```python
from build123d import *

# Parameters (mm, degrees)
SZKIC1_W                     = 53
SZKIC1_H                     = 374
SZKIC1_W_2                   = 24
SZKIC1_H_2                   = 365
DODANIE_WYCI_GNI_CIE2_DEPTH  = 12
SZKIC2_W                     = 12
SZKIC2_H                     = 3.5
WYTNIJ_WYCI_GNI_CIE1_DEPTH   = 2
SZKIC3_W                     = 53
SZKIC3_H                     = 374
DODANIE_WYCI_GNI_CIE3_DEPTH  = 2
SZKIC4_W                     = 13.3
SZKIC4_H                     = 30.500081729
SZKIC4_W_2                   = 9.4
SZKIC4_H_2                   = 64.96
WYTNIJ_WYCI_GNI_CIE2_DEPTH   = 2
SZKIC5_W                     = 2
SZKIC5_H                     = 374
DODANIE_WYCI_GNI_CIE4_DEPTH  = 43
DODANIE_WYCI_GNI_CIE5_DEPTH  = 41.5
SZKIC7_W                     = 25.5
SZKIC7_H                     = 38.500081729
DODANIE_WYCI_GNI_CIE6_DEPTH  = 1.5
SZKIC9_R                     = 12
WYTNIJ_WYCI_GNI_CIE4_DEPTH   = 1.5
DODANIE_WYCI_GNI_CIE7_DEPTH  = 43
DODANIE_WYCI_GNI_CIE8_DEPTH  = 43
SZKIC12_R                    = 12
WYTNIJ_WYCI_GNI_CIE5_DEPTH   = 1.5
SZKIC13_R                    = 9
WYTNIJ_WYCI_GNI_CIE6_DEPTH   = 1.5
SZKIC14_W                    = 57
SZKIC14_H                    = 374
SZKIC14_R                    = 12
DODANIE_WYCI_GNI_CIE9_DEPTH  = 1
SZKIC15_W                    = 57
SZKIC15_H                    = 374
SZKIC15_R                    = 12
DODANIE_WYCI_GNI_CIE10_DEPTH = 1
SZKIC16_W                    = 55
SZKIC16_H                    = 57
SZKIC16_W_2                  = 24
SZKIC16_H_2                  = 41.5
DODANIE_WYCI_GNI_CIE11_DEPTH = 1
SZKIC17_W                    = 55
SZKIC17_H                    = 57
DODANIE_WYCI_GNI_CIE12_DEPTH = 1
DODANIE_WYCI_GNI_CIE13_DEPTH = 30
SZKIC20_W                    = 55
SZKIC20_H                    = 57
DODANIE_WYCI_GNI_CIE14_DEPTH = 5.5
SZKIC21_W                    = 24
SZKIC21_H                    = 41.5
DODANIE_WYCI_GNI_CIE15_DEPTH = 5.5
SZKIC22_W                    = 57
SZKIC22_H                    = 387
SZKIC22_R                    = 12
DODANIE_WYCI_GNI_CIE16_DEPTH = 1
SZKIC23_W                    = 57
SZKIC23_H                    = 387
SZKIC23_R                    = 12
DODANIE_WYCI_GNI_CIE17_DEPTH = 1
ZAOKR_GLENIE1_R              = 1
ZAOKR_GLENIE2_R              = 1
ZAOKR_GLENIE3_R              = 1
WYTNIJ_WYCI_GNI_CIE7_DEPTH   = 0.85


with BuildPart() as part:
    # Szkic1 → Dodanie-wyciągnięcie2 (new body)
    with BuildSketch(Plane.XY):
        with Locations((-65.426891924, -133.239080048)):
            Rectangle(SZKIC1_W, SZKIC1_H)
        with Locations((-78.426891924, -133.239080048)):
            Rectangle(SZKIC1_W_2, SZKIC1_H_2, mode=Mode.SUBTRACT)
        with Locations((-52.426891924, -133.239080048)):
            Rectangle(SZKIC1_W_2, SZKIC1_H_2, mode=Mode.SUBTRACT)
    extrude(amount=DODANIE_WYCI_GNI_CIE2_DEPTH)

    # Szkic2 → Wytnij-wyciągnięcie1 (cut)
    with BuildSketch(Plane.ZY.offset(66.426891924)):
        with Locations((6, 47.510919952)):
            Rectangle(SZKIC2_W, SZKIC2_H)
    extrude(amount=-WYTNIJ_WYCI_GNI_CIE1_DEPTH, mode=Mode.SUBTRACT)

    # Szkic3 → Dodanie-wyciągnięcie3 (add)
    with BuildSketch(Plane.XY.offset(12)):
        with Locations((-65.426891924, -133.239080048)):
            Rectangle(SZKIC3_W, SZKIC3_H)
    extrude(amount=DODANIE_WYCI_GNI_CIE3_DEPTH)

    # Szkic4 → Wytnij-wyciągnięcie2 (cut)
    with BuildSketch(Plane.XY.offset(14)):
        Polygon((-46.926891924, -11.039080048), (-56.326891924, -11.039080048), (-56.326891924, -35.399080048), (-56.326891924, -40.479080048), (-46.926891924, -40.479080048), (-46.926891924, -35.399080048), align=None)
        with Locations((-47.076891924, 34.010879088)):
            Rectangle(SZKIC4_W, SZKIC4_H)
        with Locations((-83.776891924, 34.010879088)):
            Rectangle(SZKIC4_W, SZKIC4_H)
        Polygon((-74.526891924, -35.399080048), (-74.526891924, -11.039080048), (-83.926891924, -11.039080048), (-83.926891924, -35.399080048), (-83.926891924, -40.479080048), (-74.526891924, -40.479080048), align=None)
        with Locations((-51.626891924, -133.719080048)):
            Rectangle(SZKIC4_W_2, SZKIC4_H_2)
        with Locations((-79.226891924, -133.719080048)):
            Rectangle(SZKIC4_W_2, SZKIC4_H_2)
    extrude(amount=-WYTNIJ_WYCI_GNI_CIE2_DEPTH, mode=Mode.SUBTRACT)

    # Szkic5 → Dodanie-wyciągnięcie4 (add)
    with BuildSketch(Plane.XY.offset(14)):
        with Locations((-65.426891924, -133.239080048)):
            Rectangle(SZKIC5_W, SZKIC5_H)
    extrude(amount=DODANIE_WYCI_GNI_CIE4_DEPTH)

    # Szkic6 → Dodanie-wyciągnięcie5 (add)
    with BuildSketch(Plane.XY.offset(14)):
        Polygon((-64.426891924, 16.760838223), (-40.426891924, 16.760838223), (-40.426891924, 53.760919952), (-38.926891924, 53.760919952), (-38.926891924, 15.260838223), (-64.426891924, 15.260838223), align=None)
        Polygon((-90.426891924, 53.760919952), (-91.926891924, 53.760919952), (-91.926891924, 15.260838223), (-66.426891924, 15.260838223), (-66.426891924, 16.760838223), (-90.426891924, 16.760838223), align=None)
    extrude(amount=DODANIE_WYCI_GNI_CIE5_DEPTH)

    # Szkic7 → Dodanie-wyciągnięcie6 (add)
    with BuildSketch(Plane.XY.offset(55.5)):
        with Locations((-51.676891924, 34.510879088)):
            Rectangle(SZKIC7_W, SZKIC7_H)
        with Locations((-79.176891924, 34.510879088)):
            Rectangle(SZKIC7_W, SZKIC7_H)
    extrude(amount=DODANIE_WYCI_GNI_CIE6_DEPTH)

    # Szkic9 → Wytnij-wyciągnięcie4 (cut)
    with BuildSketch(Plane.ZY.offset(91.926891924)):
        with Locations((34, 34.510879088)):
            Circle(SZKIC9_R)
    extrude(amount=-WYTNIJ_WYCI_GNI_CIE4_DEPTH, mode=Mode.SUBTRACT)

    # Szkic10 → Dodanie-wyciągnięcie7 (add)
    with BuildSketch(Plane.XY.offset(14)):
        Polygon((-91.926891924, 15.260838223), (-91.926891924, -320.239080048), (-66.426891924, -320.239080048), (-66.426891924, -315.739080048), (-90.426891924, -315.739080048), (-90.426891924, 15.260838223), align=None)
    extrude(amount=DODANIE_WYCI_GNI_CIE7_DEPTH)

    # Szkic11 → Dodanie-wyciągnięcie8 (add)
    with BuildSketch(Plane.XY.offset(14)):
        Polygon((-38.926891924, 15.260838223), (-38.926891924, -320.239080048), (-64.426891924, -320.239080048), (-64.426891924, -315.739080048), (-40.426891924, -315.739080048), (-40.426891924, 15.260838223), align=None)
    extrude(amount=DODANIE_WYCI_GNI_CIE8_DEPTH)

    # Szkic12 → Wytnij-wyciągnięcie5 (cut)
    with BuildSketch(Plane(origin=(-38.926891924, 0, 0), x_dir=(0, 0, -1), z_dir=(1, 0, 0))):
        with Locations((-34, 34.510919952)):
            Circle(SZKIC12_R)
    extrude(amount=-WYTNIJ_WYCI_GNI_CIE5_DEPTH, mode=Mode.SUBTRACT)

    # Szkic13 → Wytnij-wyciągnięcie6 (cut)
    with BuildSketch(Plane.XY.offset(57)):
        with Locations((-78.426891924, 32.810879088)):
            Circle(SZKIC13_R)
        with Locations((-52.426891924, 32.810879088)):
            Circle(SZKIC13_R)
    extrude(amount=-WYTNIJ_WYCI_GNI_CIE6_DEPTH, mode=Mode.SUBTRACT)

    # Szkic14 → Dodanie-wyciągnięcie9 (add)
    with BuildSketch(Plane(origin=(-38.926891924, 0, 0), x_dir=(0, 0, -1), z_dir=(1, 0, 0))):
        with Locations((-28.5, -133.239080048)):
            Rectangle(SZKIC14_W, SZKIC14_H)
        with Locations((-34, 34.510919952)):
            Circle(SZKIC14_R, mode=Mode.SUBTRACT)
    extrude(amount=DODANIE_WYCI_GNI_CIE9_DEPTH)

    # Szkic15 → Dodanie-wyciągnięcie10 (add)
    with BuildSketch(Plane.ZY.offset(91.926891924)):
        with Locations((28.5, -133.239080048)):
            Rectangle(SZKIC15_W, SZKIC15_H)
        with Locations((34, 34.510879088)):
            Circle(SZKIC15_R, mode=Mode.SUBTRACT)
    extrude(amount=DODANIE_WYCI_GNI_CIE10_DEPTH)

    # Szkic16 → Dodanie-wyciągnięcie11 (add)
    with BuildSketch(Plane(origin=(0, 53.760919952, 0), x_dir=(1, 0, 0), z_dir=(0, 1, 0))):
        with Locations((-65.426891924, -28.5)):
            Rectangle(SZKIC16_W, SZKIC16_H)
        with Locations((-52.426891924, -34.75)):
            Rectangle(SZKIC16_W_2, SZKIC16_H_2, mode=Mode.SUBTRACT)
        with Locations((-78.426891924, -34.75)):
            Rectangle(SZKIC16_W_2, SZKIC16_H_2, mode=Mode.SUBTRACT)
    extrude(amount=DODANIE_WYCI_GNI_CIE11_DEPTH)

    # Szkic17 → Dodanie-wyciągnięcie12 (add)
    with BuildSketch(Plane.XZ.offset(320.239080048)):
        with Locations((-65.426891924, 28.5)):
            Rectangle(SZKIC17_W, SZKIC17_H)
    extrude(amount=DODANIE_WYCI_GNI_CIE12_DEPTH)

    # Szkic18 → Dodanie-wyciągnięcie13 (add)
    with BuildSketch(Plane.XY.offset(57)):
        Polygon((-64.426891924, 15.260838223), (-64.426891924, 54.760919952), (-66.426891924, 54.760919952), (-66.426891924, 15.260838223), (-66.426891924, -4.739161777), (-66.426891924, -24.739161777), (-64.426891924, -24.739161777), (-64.426891924, -4.739161777), align=None)
    extrude(amount=DODANIE_WYCI_GNI_CIE13_DEPTH)

    # Szkic20 → Dodanie-wyciągnięcie14 (add)
    with BuildSketch(Plane.XZ.offset(321.239080048)):
        with Locations((-65.426891924, 28.5)):
            Rectangle(SZKIC20_W, SZKIC20_H)
    extrude(amount=DODANIE_WYCI_GNI_CIE14_DEPTH)

    # Szkic21 → Dodanie-wyciągnięcie15 (add)
    with BuildSketch(Plane(origin=(0, 54.760919952, 0), x_dir=(1, 0, 0), z_dir=(0, 1, 0))):
        Polygon((-64.426891924, -87), (-66.426891924, -87), (-66.426891924, -57), (-92.926891924, -57), (-92.926891924, 0), (-37.926891924, 0), (-37.926891924, -57), (-64.426891924, -57), align=None)
        with Locations((-52.426891924, -34.75)):
            Rectangle(SZKIC21_W, SZKIC21_H, mode=Mode.SUBTRACT)
        with Locations((-78.426891924, -34.75)):
            Rectangle(SZKIC21_W, SZKIC21_H, mode=Mode.SUBTRACT)
    extrude(amount=DODANIE_WYCI_GNI_CIE15_DEPTH)

    # Szkic22 → Dodanie-wyciągnięcie16 (add)
    with BuildSketch(Plane(origin=(-37.926891924, 0, 0), x_dir=(0, 0, -1), z_dir=(1, 0, 0))):
        with Locations((-28.5, -133.239080048)):
            Rectangle(SZKIC22_W, SZKIC22_H)
        with Locations((-34, 34.510919952)):
            Circle(SZKIC22_R, mode=Mode.SUBTRACT)
    extrude(amount=DODANIE_WYCI_GNI_CIE16_DEPTH)

    # Szkic23 → Dodanie-wyciągnięcie17 (add)
    with BuildSketch(Plane.ZY.offset(92.926891924)):
        with Locations((28.5, -133.239080048)):
            Rectangle(SZKIC23_W, SZKIC23_H)
        with Locations((34, 34.510879088)):
            Circle(SZKIC23_R, mode=Mode.SUBTRACT)
    extrude(amount=DODANIE_WYCI_GNI_CIE17_DEPTH)

    # Zaokrąglenie1
    zaokr_glenie1_edges = [part.edges().sort_by_distance(p)[0] for p in [
        (-65.426891924, -24.739161777, 87),
    ]]
    fillet(zaokr_glenie1_edges, radius=ZAOKR_GLENIE1_R)

    # Zaokrąglenie2
    zaokr_glenie2_edges = [part.edges().sort_by_distance(p)[0] for p in [
        (-65.426891924, -24.739161777, 57),
    ]]
    fillet(zaokr_glenie2_edges, radius=ZAOKR_GLENIE2_R)

    # Zaokrąglenie3
    zaokr_glenie3_edges = [part.edges().sort_by_distance(p)[0] for p in [
        (-65.426891924, 60.260919952, 87),
    ]]
    fillet(zaokr_glenie3_edges, radius=ZAOKR_GLENIE3_R)

    # Szkic24 → Wytnij-wyciągnięcie7 (cut)
    with BuildSketch(Plane.XY.offset(57)):
        Polygon((-64.426891924, 15.260838223), (-64.426891924, -25.739161777), (-66.426891924, -25.739161777), (-66.426891924, 15.260838223), (-93.926891924, 15.260838223), (-93.926891924, -326.739080048), (-36.926891924, -326.739080048), (-36.926891924, 15.260838223), align=None)
    extrude(amount=-WYTNIJ_WYCI_GNI_CIE7_DEPTH, mode=Mode.SUBTRACT)


solid = part.part
```
Work out the finished part from the listing and answer in its coordinate system (mm). A direction names the side the tool comes from. Give positions to 0.01 mm unless a question says otherwise; leave off trailing zeros. Loops run counter-clockwise (first coordinate to the right, second up) from the corner with the lowest first, then second, coordinate; pieces in that order, holes last. Notation, with made-up numbers: (69, 80) -> (110, 80) arc R8 cw to (110, 86) -> close; hole circle Ø10 at (57, -10.5). An arc over 180 degrees is marked (long way). Write item = value, one per line. Start each with the question number.
(1) Find section D-D on z = 73. Give the vertices of the cut face in (x, y).
(2) Find section B-B on z = 34. Give the vertices of the cut face in (x, y), and give its area (4 significant figures).
(3) Given pin 1 Ø6 at (y, z) = (-239, 59) entering from -X; pin 2 Ø12 at (x, y) = (-81, 48) entering from +Z; pin 3 Ø2 at (x, z) = (-82.5, 19.5) entering from +Y; pin 4 Ø12 at (x, y) = (-57.5, 29.5) entering from -Z, each flat-ended and moving along its own axis, determine where each tip first touches the part or whether it passes through.
(4) Find section A-A on y = -141. Give the vertices of the cut face in (x, z), and give its area (3 significant figures).
(5) Find section C-C on y = -74. Give the vertices of the cut face in (x, z), and give its area (3 significant figures).
(6) The mould has two halves that part along Y. Classify faces 5 (the flat face through (-58, 43, 14)), 6 (the flat face through (-53, 16.761, 34)), 7 (the flat face through (-40.427, -153, 35)): +Y half, -Y half, draft (parallel to the pull), parting line (faces both ways), or undercut.
(7) Which of the six approach directions +Z, -Z, +X, -X, +Y, -Y give full straight-line access (tool end or side, diameter ignored) to faces 1 (the flat face through (-79, 43, 55.5)), 2 (the flat face through (-64.427, -130, 42)), 3 (the flat face through (-80, 42, 57)), 4 (the flat face through (-66, 49.261, 7))?
(8) Find the intervals of material crossed by probe 1 along X at (y, z) = (-228.5, 35); probe 2 along Y at (x, z) = (-42, 13); probe 3 along Y at (x, z) = (-88.5, 27.5), in increasing order. Write a range as from..to.
From the geometry:
q1.outline = (-66.43, -24.74) -> (-64.43, -24.74) -> (-64.43, 60.26) -> (-66.43, 60.26) -> close
q2.outline = (-93.93, -326.74) -> (-36.93, -326.74) -> (-36.93, 22.51) -> (-40.43, 22.51) -> (-40.43, 16.76) -> (-64.43, 16.76) -> (-64.43, 60.26) -> (-66.43, 60.26) -> (-66.43, 16.76) -> (-90.43, 16.76) -> (-90.43, 22.51) -> (-93.93, 22.51) -> close; (-93.93, 46.51) -> (-90.43, 46.51) -> (-90.43, 60.26) -> (-93.93, 60.26) -> close; (-40.43, 46.51) -> (-36.93, 46.51) -> (-36.93, 60.26) -> (-40.43, 60.26) -> close; hole (-90.43, -315.74) -> (-66.43, -315.74) -> (-66.43, 15.26) -> (-90.43, 15.26) -> close; hole (-64.43, -315.74) -> (-40.43, -315.74) -> (-40.43, 15.26) -> (-64.43, 15.26) -> close
q2.area = 3,915 mm^2
q3.pin_1 = -93.93
q3.pin_2 = 57
q3.pin_3 = 16.76
q3.pin_4 = 12
q4.outline = (-93.93, 0) -> (-90.43, 0) -> (-90.43, 12) -> (-83.93, 12) -> (-83.93, 14) -> (-90.43, 14) -> (-90.43, 56.15) -> (-93.93, 56.15) -> close; (-74.53, 12) -> (-66.43, 12) -> (-66.43, 0) -> (-64.43, 0) -> (-64.43, 12) -> (-56.33, 12) -> (-56.33, 14) -> (-64.43, 14) -> (-64.43, 56.15) -> (-66.43, 56.15) -> (-66.43, 14) -> (-74.53, 14) -> close; (-46.93, 12) -> (-40.43, 12) -> (-40.43, 0) -> (-36.93, 0) -> (-36.93, 56.15) -> (-40.43, 56.15) -> (-40.43, 14) -> (-46.93, 14) -> close
q4.area = 564 mm^2
q5.outline = (-93.93, 0) -> (-90.43, 0) -> (-90.43, 12) -> (-66.43, 12) -> (-66.43, 0) -> (-64.43, 0) -> (-64.43, 12) -> (-40.43, 12) -> (-40.43, 0) -> (-36.93, 0) -> (-36.93, 56.15) -> (-40.43, 56.15) -> (-40.43, 14) -> (-64.43, 14) -> (-64.43, 56.15) -> (-66.43, 56.15) -> (-66.43, 14) -> (-90.43, 14) -> (-90.43, 56.15) -> (-93.93, 56.15) -> close
q5.area = 601 mm^2
q6.face_5 = draft
q6.face_6 = +Y half
q6.face_7 = undercut
q7.face_1 = +Y
q7.face_2 = +Z
q7.face_3 = +Z, -X, +Y, -Y
q7.face_4 = -Z
q8.probe_1 = -93.93..-90.43, -66.43..-64.43, -40.43..-36.93
q8.probe_2 = -326.74..18.76, 49.26..60.26
q8.probe_3 = -326.74..-315.74, 15.26..16.76
